Autodesk Inventor part; units mm, degrees
ref_plane "YZ Plane" through (0, 0, 0) normal (1, 0, 0) x (0, 1, 0)
ref_plane "XZ Plane" through (0, 0, 0) normal (0, 1, 0) x (-1, 0, 0)
ref_plane "XY Plane" through (0, 0, 0) normal (0, 0, 1) x (1, 0, 0)
sketch "Sketch1" plane through (0, 0, 0) normal (0, 1, 0) x (-1, 0, 0)
  line L0 (-50.5, 29.5) -> (50.5, 29.5)
  line L1 (50.5, 29.5) -> (50.5, -29.5)
  line L2 (50.5, -29.5) -> (-50.5, -29.5)
  line L3 (-50.5, -29.5) -> (-50.5, 29.5)
  line L4 (-50.5, 29.5) -> (50.5, -29.5) construction
  line L5 (50.5, 29.5) -> (-50.5, -29.5) construction
  line L6 (5.5, 16.6667) -> (10.5, 16.6667)
  line L7 (10.5, 6.6667) -> (5.5, 6.6667)
  line L8 (5.5, 6.6667) -> (5.5, 16.6667)
  line L9 (5.5, 16.6667) -> (10.5, 6.6667) construction
  line L10 (10.5, 16.6667) -> (5.5, 6.6667) construction
  line L11 (5.5, -6.6667) -> (10.5, -6.6667)
  line L12 (10.5, -16.6667) -> (5.5, -16.6667)
  line L13 (5.5, -16.6667) -> (5.5, -6.6667)
  line L14 (5.5, -6.6667) -> (10.5, -16.6667) construction
  line L15 (10.5, -6.6667) -> (5.5, -16.6667) construction
  line L16 (10.5, 10) -> (20.5, 10)
  line L17 (20.5, 11) -> (20.5, 9)
  line L18 (20.5, 9) -> (10.5, 9)
  line L19 (20.5, 11) -> (10.5, 11)
  line L20 (48.5, 27.5) -> (20.5, 27.5)
  line L21 (20.5, 27.5) -> (20.5, -27.5)
  line L22 (20.5, -27.5) -> (48.5, -27.5)
  line L23 (48.5, -27.5) -> (48.5, 27.5)
  line L24 (10.5, 16.6667) -> (10.5, 13.3333)
  line L25 (10.5, 13.3333) -> (10.5, 10)
  line L26 (10.5, 10) -> (10.5, 6.6667)
  line L27 (10.5, -16.6667) -> (10.5, -13.3333)
  line L28 (10.5, -13.3333) -> (10.5, -10)
  line L29 (10.5, -10) -> (10.5, -6.6667)
  line L30 (8, -11.6667) -> (8, 11.6667)
  line L31 (-50.5, 0) -> (50.5, 0)
  point P0 (0, 0)
  point P1 (0, 29.5)
  point P2 (0, -29.5)
  point P3 (0, 0)
  point P4 (8, 0)
  dimension "d0" = 101
  dimension "d1" = 59
  dimension "d7" = 5
  dimension "d8" = 10
  dimension "d9" = 5
  dimension "d10" = 10
  dimension "d11" = 10
  dimension "d12" = 2
  dimension "d16" = 2
  dimension "d17" = 2
  dimension "d18" = 2
  dimension "d19" = 28
  dimension "d20" = 20
extrude "Extrusion2" add sketch "Sketch1" along normal blind 3 contours L0 L1 L31 L23 L20 L21 L19 L25 L24 L6 L8 L7 L30 L3 | L31 L21 L22 L23 L1 L2 L3 | L30 L7 L26 L18 L21 L31
properties part number "Lag 3"
Check sheet for the modelled part. Datum: model origin and axes. Units: mm. A direction names the side the tool comes from. Round coordinates to 2 decimals unless told otherwise and drop trailing zeros. Order: outer loops, then holes, each group sorted by start corner. A loop starts at its lowest first (then second) coordinate and runs counter-clockwise, first axis right, second up. Notation, with made-up numbers: M 87,74 L 142,74 A32 ccw 142,113 Z; hole C 21.5,20 d2. An arc over 180 degrees is marked long. Answer in a Markdown table with one row per item.
(1) Section check A-A on x = -12.5. Record the boundary of the cut face in (y, z), plus the area to 3 significant figures.
Findings:
| item | result |
|---|---|
| outline | M 0,-29.5 L 3,-29.5 L 3,9 L 0,9 Z; M 0,11 L 3,11 L 3,29.5 L 0,29.5 Z |
| area | 171 mm^2 |
(2) Section check D-D on z = -8. Record the boundary of the cut face in (x, y).
Findings:
| item | result |
|---|---|
| outline | M -50.5,0 L -48.5,0 L -48.5,3 L -50.5,3 Z; M -20.5,0 L -10.5,0 L -10.5,3 L -20.5,3 Z; M -5.5,0 L 50.5,0 L 50.5,3 L -5.5,3 Z |
(3) Set-up check for faces 1 (the flat face through (-5.5, 1, 12)), 2 (the flat face through (12, 0, 0)): record each of +Z, -Z, +X, -X, +Y, -Y from which the full face is reachable in a straight line by a thin tool's end or side.
Findings:
| item | result |
|---|---|
| face 1 | +Y, -Y |
| face 2 | +Z, -Z, +X, -X, -Y |
(4) Section check B-B on y = 1.2. Record the boundary of the cut face in (x, z), plus the area to 3 significant figures.
Findings:
| item | result |
|---|---|
| outline | M -50.5,-29.5 L 50.5,-29.5 L 50.5,29.5 L -50.5,29.5 Z; hole M -48.5,-27.5 L -20.5,-27.5 L -20.5,9 L -10.5,9 L -10.5,6.67 L -5.5,6.67 L -5.5,16.67 L -10.5,16.67 L -10.5,11 L -20.5,11 L -20.5,27.5 L -48.5,27.5 Z; hole M -10.5,-16.67 L -5.5,-16.67 L -5.5,-6.67 L -10.5,-6.67 Z |
| area | 4,300 mm^2 |
(5) Section check C-C on z = 3.5. Record the boundary of the cut face in (x, y).
Findings:
| item | result |
|---|---|
| outline | M -50.5,0 L -48.5,0 L -48.5,3 L -50.5,3 Z; M -20.5,0 L 50.5,0 L 50.5,3 L -20.5,3 Z |
(6) Draft check along X on faces 3 (the flat face through (1, 1, 29.5)), 4 (the flat face through (-8, 1, 16.667)), 5 (the flat face through (-50.5, 1, 0)). Enter one of: +X half, -X half, draft (parallel to the pull), parting line (faces both ways), or undercut.
Findings:
| item | result |
|---|---|
| face 3 | draft |
| face 4 | undercut |
| face 5 | -X half |
(7) Material ranges on line 1 along Z through (x, y) = (-10, 1.1); line 2 along X through (y, z) = (2.45, 8.5); line 3 along Z through (x, y) = (-18.5, 2.55), recorded low to high. Write a range as from..to.
Findings:
| item | result |
|---|---|
| line 1 | z = -29.5..-16.67, -6.67..6.67, 16.67..29.5 |
| line 2 | x = -50.5..-48.5, -20.5..-10.5, -5.5..50.5 |
| line 3 | z = -29.5..9, 11..29.5 |
